```python
from build123d import *

# Parameters (mm, degrees)
BOSS_EXTRUDE1_DEPTH = 10
SKETCH2_R           = 1.5
CUT_EXTRUDE1_DEPTH  = 5
CIRPATTERN1_COUNT   = 3


with BuildPart() as part:
    # Sketch1 → Boss-Extrude1 (new body)
    with BuildSketch(Plane.XY):
        Polygon((86.602540378, 0), (43.301270189, 75), (-43.301270189, 75), (-86.602540378, 0), (-43.301270189, -75), (43.301270189, -75), align=None)
    extrude(amount=BOSS_EXTRUDE1_DEPTH)

    # Sketch2 → Cut-Extrude1 (cut)
    with BuildSketch(Plane.XZ.offset(75)):
        with Locations((-10, 5)):
            Circle(SKETCH2_R)
        with Locations((10, 5)):
            Circle(SKETCH2_R)
    cut_extrude1 = extrude(amount=-CUT_EXTRUDE1_DEPTH, mode=Mode.SUBTRACT)

    # CirPattern1: Cut-Extrude1 ×3 about axis
    cirpattern1_axis = Axis((0, 0, 0), (0, 0, 1))
    for i in range(1, CIRPATTERN1_COUNT):
        add(cut_extrude1.rotate(cirpattern1_axis, i * 360 / CIRPATTERN1_COUNT), mode=Mode.SUBTRACT)


solid = part.part
```
For this review, take the finished solid that the model builds, in its own axes (mm). Give positions to 0.01 mm unless a question says otherwise; leave off trailing zeros. Write each loop counter-clockwise with the first axis right and the second up, starting at its lowest first coordinate (ties: lowest second). Pieces come first, ordered by that corner, then holes.
Item 1: The part is to be moulded in two halves that separate along Z. For faces 1 (the face through (-64.65, 38.02, 4.93)), 2 (the face through (-1, 1, 10)), 3 (the face through (-68.533, 26.368, 5.451)), say which applies: +Z half, -Z half, draft (parallel to the pull), parting line (faces both ways), or undercut.
Item 2: Take a section at B-B (y = -50.5). Give the boundary of the cut face in (x, z), and give its area (3 significant figures).
Item 3: Take a section at C-C (x = 47.5). Give the boundary of the cut face in (y, z), and give its area (3 significant figures).
Item 4: Insertion check: P1, Ø0.9, axis at x = -10.5, z = 5, coming from the -Y side; P2, Ø6, axis at y = 36.5, z = 1.5, coming from the +X side; P3, Ø5, axis at y = 52.5, z = 6, coming from the +X side (3 decimals). Each pin has a flat end and moves straight along its axis. Give the tip position at first contact, or say it passes through.
Item 5: Wall thickness on probe 1 along Z at (x, y) = (10, -73); probe 2 along X at (y, z) = (27.5, 1.5); probe 3 along X at (y, z) = (-37, 4.75): over which ranges is each line inside the solid? List them lowest first.
Established:
1. face 1: draft
1. face 2: +Z half
1. face 3: undercut
2. outline: (-57.45, 0) - (57.45, 0) - (57.45, 10) - (-57.45, 10) - close
2. area: 1,150 mm2
3. outline: (-67.73, 0) - (67.73, 0) - (67.73, 10) - (-67.73, 10) - close
3. area: 1,350 mm2
4. P1: stops at y = -70
4. P2: stops at x = 67.26
4. P3: stops at x = 57.735
5. probe 1: z = 0 to 3.5, 6.5 to 10
5. probe 2: x = -70.73 to 70.73
5. probe 3: x = -65.24 to 65.24
